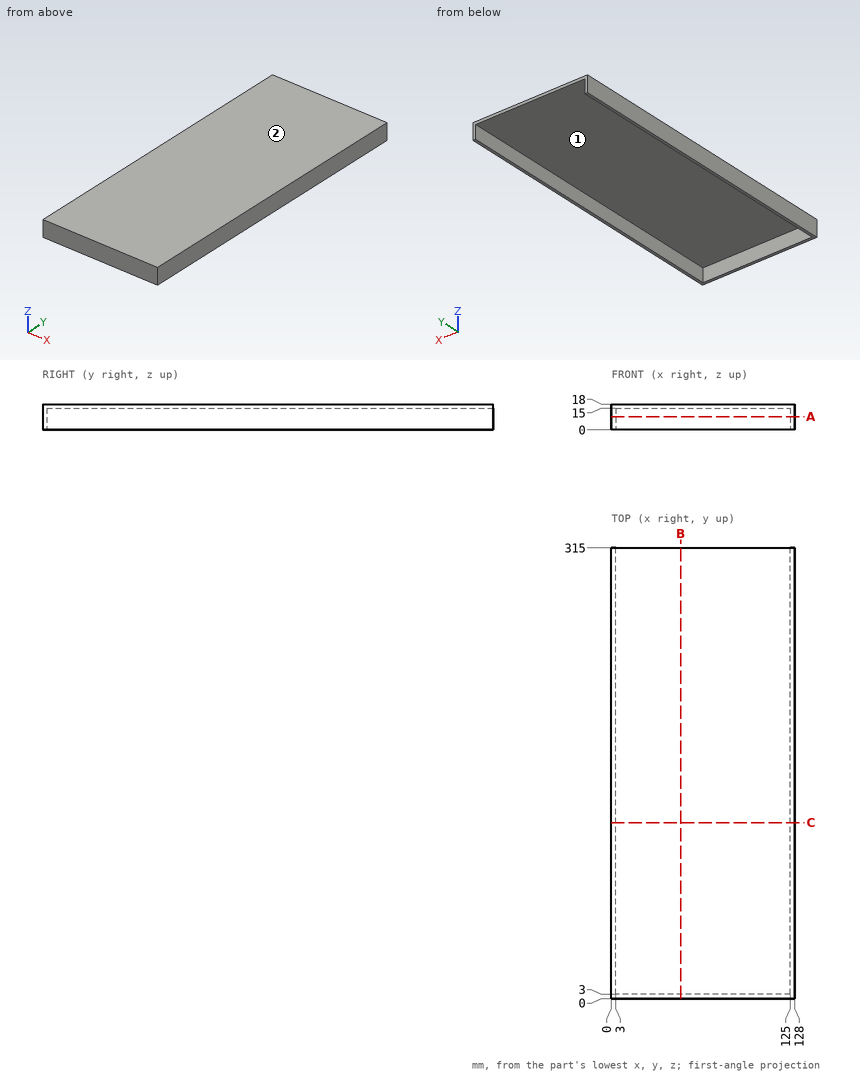
Verification items for this drawing (mm, ordinates from the low corner). Coordinates: 2 decimals unless noted, no trailing zeros. Write each loop counter-clockwise with the first axis right and the second up, starting at its lowest first coordinate (ties: lowest second). Pieces come first, ordered by that corner, then holes. Notation, with made-up numbers: M -0.75,41.25 L 15.25,41.25 A21 ccw 15.25,58.25 Z; hole C 27.5,-38 d1. An arc over 180 degrees is marked long. One line per item, written item: value. Start each with the question number.
(1) Release check for a two-part mould opening along X. For the marked faces 1 and 2 record: released by +X, released by -X, zero draft, split by the parting line, or undercut.
(2) Sectioned sample at C-C, the plane y = 123. Enter the section's corners in (x, z).
(3) Sectioned sample at B-B, the plane x = 48.5. Enter the section's corners in (y, z), and give its area (3 significant figures).
(4) Scan lines: line 1 along X through (y, z) = (141, 4.25); line 2 along Y through (x, z) = (35, 12.5); line 3 along Z through (x, y) = (57, 136). Record each from-to range of solid material in increasing order. Write a range as [from, to].
(5) Depth check by flat-ended pin: pin 1 (1 mm diameter, centred on x = 80, z = 5, fed in from +Y); pin 2 (10 mm diameter, centred on y = 84, z = 3, fed in from -X); pin 3 (6 mm diameter, centred on x = 56, y = 42.5, fed in from -Z). Enter the tip coordinate at first touch or a pass-through.
(6) Sectioned sample at A-A, the plane z = 9.25. Enter the section's corners in (x, y).
Filled sheet:
1. face 1: undercut
1. face 2: zero draft
2. outline: M 0,0 L 3,0 L 3,15 L 125,15 L 125,0 L 128,0 L 128,18 L 0,18 Z
3. outline: M 0,0 L 3,0 L 3,15 L 315,15 L 315,18 L 0,18 Z
3. area: 990 mm²
4. line 1: [0, 3], [125, 128]
4. line 2: [0, 3]
4. line 3: [15, 18]
5. pin 1: y = 3
5. pin 2: x = 0
5. pin 3: z = 15
6. outline: M 0,0 L 128,0 L 128,315 L 125,315 L 125,3 L 3,3 L 3,315 L 0,315 Z
